Could you check a few things on this model? Use its own coordinates, in mm. Give positions to 0.01 mm unless a question says otherwise; leave off trailing zeros. Order: outer loops, then holes, each group sorted by start corner. A loop starts at its lowest first (then second) coordinate and runs counter-clockwise, first axis right, second up.
from build123d import *

# Parameters (mm, degrees)
SKETCH1_W               = 158.76
SKETCH1_H               = 146.36
BOSS_EXTRUDE1_DEPTH     = 3.18
CUT_EXTRUDE1_START      = -4.18
SKETCH2_W               = 29.94
SKETCH2_H               = 3.18
SKETCH2_W_2             = 59.38
CUT_EXTRUDE1_DEPTH      = 5.18
CUT_EXTRUDE2_START      = -4.18
SKETCH3_R               = 1.55
CUT_EXTRUDE2_DEPTH      = 5.18
MIRROR3_START           = -4.18
MIRROR3_COPY_1_SKETCH_R = 1.55
MIRROR3_COPY_1_DEPTH    = 5.18
CUT_EXTRUDE3_START      = -4.18
SKETCH5_W               = 3.18
SKETCH5_H               = 20
SKETCH5_W_2             = 2.82
SKETCH5_H_2             = 7
SKETCH5_W_3             = 13
SKETCH5_H_3             = 3
CUT_EXTRUDE3_DEPTH      = 5.18
SKETCH7_R               = 1.6
CUT_EXTRUDE4_DEPTH      = 1
CUT_EXTRUDE4_DEPTH_BACK = 4.18


with BuildPart() as part:
    # Sketch1 → Boss-Extrude1 (new body)
    with BuildSketch(Plane.XY):
        Rectangle(SKETCH1_W, SKETCH1_H)
    extrude(amount=BOSS_EXTRUDE1_DEPTH)

    # Sketch2 → Cut-Extrude1 (cut)
    with BuildSketch(Plane.XY.offset(3.18).offset(CUT_EXTRUDE1_START)):
        with Locations((-64.41, 71.59)):
            Rectangle(SKETCH2_W, SKETCH2_H)
        with Locations((0, 71.59)):
            Rectangle(SKETCH2_W_2, SKETCH2_H)
        with Locations((64.41, 71.59)):
            Rectangle(SKETCH2_W, SKETCH2_H)
    cut_extrude1 = extrude(amount=CUT_EXTRUDE1_DEPTH, mode=Mode.SUBTRACT)

    # Mirror1: Cut-Extrude1 across plane
    add(cut_extrude1.mirror(Plane.ZX), mode=Mode.SUBTRACT)

    # Sketch3 → Cut-Extrude2 (cut)
    with BuildSketch(Plane.XY.offset(3.18).offset(CUT_EXTRUDE2_START)):
        with Locations((-39.565, -71.18)):
            Circle(SKETCH3_R)
    cut_extrude2 = extrude(amount=CUT_EXTRUDE2_DEPTH, mode=Mode.SUBTRACT)

    # Mirror2: Cut-Extrude2 across plane
    add(cut_extrude2.mirror(Plane(origin=(0, 0, 0), x_dir=(0, 0, 1), z_dir=(1, 0, 0))), mode=Mode.SUBTRACT)

    # Mirror3: Cut-Extrude2 across plane
    add(cut_extrude2.mirror(Plane.ZX), mode=Mode.SUBTRACT)

    # Mirror3 copy 1 sketch → Mirror3 copy 1 (cut)
    with BuildSketch(Plane(origin=(0, 0, 3.18), x_dir=(-1, 0, 0), z_dir=(0, 0, 1)).offset(MIRROR3_START)):
        with Locations((-39.565, -71.18)):
            Circle(MIRROR3_COPY_1_SKETCH_R)
    extrude(amount=MIRROR3_COPY_1_DEPTH, mode=Mode.SUBTRACT)

    # Sketch5 → Cut-Extrude3 (cut)
    with BuildSketch(Plane(origin=(0, 0, 0), x_dir=(-1, 0, 0), z_dir=(0, 0, -1)).offset(CUT_EXTRUDE3_START)):
        with Locations((-77.79, 0)):
            Rectangle(SKETCH5_W, SKETCH5_H)
        with Locations((-70.79, 0)):
            Rectangle(SKETCH5_W_2, SKETCH5_H_2)
        with Locations((-72.88, 0)):
            Rectangle(SKETCH5_W_3, SKETCH5_H_3)
    cut_extrude3 = extrude(amount=CUT_EXTRUDE3_DEPTH, mode=Mode.SUBTRACT)

    # Mirror4: Cut-Extrude3 across plane
    add(cut_extrude3.mirror(Plane(origin=(0, 0, 0), x_dir=(0, 0, 1), z_dir=(1, 0, 0))), mode=Mode.SUBTRACT)

    # Sketch7 → Cut-Extrude4 (cut, two sides)
    with BuildSketch(Plane(origin=(0, 0, 0), x_dir=(-1, 0, 0), z_dir=(0, 0, -1))) as cut_extrude4_sk:
        with Locations((64.474463585, 48.325)):
            Circle(SKETCH7_R)
        with Locations((16.174463585, 49.925)):
            Circle(SKETCH7_R)
        with Locations((49.174463585, -2.475)):
            Circle(SKETCH7_R)
        with Locations((21.274463585, -2.475)):
            Circle(SKETCH7_R)
    extrude(amount=CUT_EXTRUDE4_DEPTH, mode=Mode.SUBTRACT)
    extrude(cut_extrude4_sk.sketch, amount=-CUT_EXTRUDE4_DEPTH_BACK, mode=Mode.SUBTRACT)


solid = part.part
Item 1: Please list where these lines run through material, in increasing order: line 1 along Y through (x, z) = (59.5, 0.7); line 2 along X through (y, z) = (-5, 3); line 3 along Y through (x, z) = (-40.5, 1.65).
Findings:
line 1: y = -70 to 70
line 2: x = -76.2 to 76.2
line 3: y = -73.18 to -72.42, -69.94 to 69.94, 72.42 to 73.18
Item 2: For pin 1 (1 mm diameter, centred on y = -2, z = 2, fed in from -X); pin 2 (1 mm diameter, centred on x = -1.5, z = 1.5, fed in from +Y); pin 3 (0.9 mm diameter, centred on x = 68, z = 2, fed in from -Y), each with a flat end and sliding along its axis, tell me the tip position at first contact or that it passes through.
Findings:
pin 1: stops at x = -76.2
pin 2: stops at y = 70
pin 3: stops at y = -70
Item 3: Imagine slicing it at B-B on y = 6. List the corners of the cut face in (x, z) for me.
Findings:
outline: (-76.2, 0) - (76.2, 0) - (76.2, 3.18) - (-76.2, 3.18) - close
Item 4: Imagine slicing it at A-A on x = 24.5. List the corners of the cut face in (y, z) for me, then the cut area to 3 significant figures.
Findings:
outline: (-70, 0) - (70, 0) - (70, 3.18) - (-70, 3.18) - close
area: 445 mm2
Item 5: Imagine slicing it at C-C on z = 1.8. Give the number of separate pieces and of enclosed holes in the cut face, then the cut area to 3 significant figures.
Findings:
separate pieces: 1
enclosed holes: 8
area: 22,200 mm2
